from build123d import *

# Parameters (mm, degrees)
F0_W     = 25.4
F0_H     = 33.528
F1_DEPTH = 5.715
F3_W     = 20.066
F3_H     = 33.655
F4_DEPTH = 5.08
F5_W     = 20.066
F5_H     = 8.89
F6_DEPTH = 25.4


with BuildPart() as f1:
    # F0 (on Top) → F1 (new body)
    with BuildSketch(Plane.XY):
        Rectangle(F0_W, F0_H)
    extrude(amount=F1_DEPTH)

    # F3 (on face) → F4 (cut)
    with BuildSketch(Plane.XY.offset(5.715)):
        Rectangle(F3_W, F3_H)
    extrude(amount=-F4_DEPTH, mode=Mode.SUBTRACT)

    # F5 (on face) → F6 (cut)
    with BuildSketch(Plane.XY.offset(0.635)):
        with Locations((0, -12.319)):
            Rectangle(F5_W, F5_H)
    extrude(amount=-F6_DEPTH, mode=Mode.SUBTRACT)


solid = f1.part
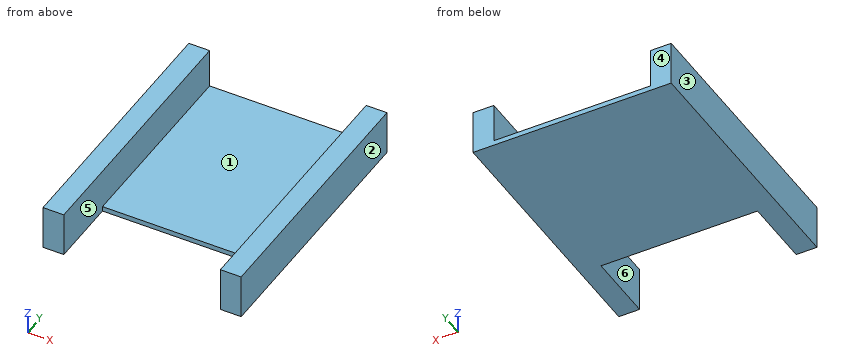
Could you check a few things on this model? Use its own coordinates, in mm. Face numbers are marked on the shaded views. A direction names the side the tool comes from. Round coordinates to 2 decimals unless told otherwise and drop trailing zeros. Loops run counter-clockwise (first coordinate to the right, second up) from the corner with the lowest first, then second, coordinate; pieces in that order, holes last. Notation, with made-up numbers: (80.5, 2) -> (92.5, 2) arc R12 ccw to (92.5, 17) -> close; hole circle Ø1 at (73.5, 80.5). An arc over 180 degrees is marked (long way). Use CSV: the item, a comma, the result in double quotes.
(1) For the marked faces 1 and 2, which set-ups out of +Z, -Z, +X, -X, +Y, -Y let a thin tool reach every point of the face, with its end or its side?
Return value:
face 1,"+Z, +Y, -Y"
face 2,"+Z, -Z, +X, +Y, -Y"
(2) Will these pins go through, and if not, where does the flat tip stop? pin 1 Ø8 at (x, y) = (2, -3) entering from +Z (3 decimals); pin 2 Ø0.5 at (x, z) = (4.5, 0.5) entering from -Y.
Return value:
pin 1,"stops at z = 0.635"
pin 2,"stops at y = -7.87"
(3) Suppose I cut it at B-B on y = 1. Write out the boundary of the cut face in (x, z) (3 decimals).
Return value:
outline,"(-12.7, 0) -> (12.7, 0) -> (12.7, 5.715) -> (10.033, 5.715) -> (10.033, 0.635) -> (-10.033, 0.635) -> (-10.033, 5.715) -> (-12.7, 5.715) -> close"
(4) If we mould it in two halves opening along X, with no side actions, what happens to the marked faces 3, 4, 5 and 6? For each: +X half, -X half, draft (parallel to the pull), parting line (faces both ways), or undercut.
Return value:
face 3,"-X half"
face 4,"draft"
face 5,"undercut"
face 6,"undercut"
(5) If I drill on probe 1 along X at (y, z) = (-1.5, 2); probe 2 along Z at (x, y) = (-9, 15) (3 decimals); probe 3 along Y at (x, z) = (-2.5, 0.5), over which ranges is the centre line in solid material (lowest first)? Write a range as [from, to].
Return value:
probe 1,"x = [-12.7, -10.03], [10.03, 12.7]"
probe 2,"z = [0, 0.635]"
probe 3,"y = [-7.87, 16.76]"
(6) Suppose I cut it at C-C on x = -2.5. Write out the boundary of the cut face in (y, z) (3 decimals).
Return value:
outline,"(-7.874, 0) -> (16.764, 0) -> (16.764, 0.635) -> (-7.874, 0.635) -> close"
(7) Suppose I cut it at A-A on z = 1.3. Write out the boundary of the cut face in (x, y).
Return value:
outline,"(-12.7, -16.76) -> (-10.03, -16.76) -> (-10.03, 16.76) -> (-12.7, 16.76) -> close; (10.03, -16.76) -> (12.7, -16.76) -> (12.7, 16.76) -> (10.03, 16.76) -> close"
